from build123d import *

# Parameters (mm, degrees)
SKETCH1_W           = 5
SKETCH1_H           = 70
BOSS_EXTRUDE1_DEPTH = 10


with BuildPart() as part:
    # Sketch1 → Boss-Extrude1 (new body)
    with BuildSketch(Plane.XY):
        Polygon((-124.392981478, -115.783921891), (0, -115.783921891), (124.407018522, -115.783921891), (124.407018522, -15.783921891), (-0.05047515, -15.783921891), (-124.392981478, -15.783921891), align=None)
        with Locations((-31.092981478, -55.783921891)):
            Rectangle(SKETCH1_W, SKETCH1_H, mode=Mode.SUBTRACT)
        with Locations((-93.292981478, -55.783921891)):
            Rectangle(SKETCH1_W, SKETCH1_H, mode=Mode.SUBTRACT)
        with Locations((31.107018522, -55.783921891)):
            Rectangle(SKETCH1_W, SKETCH1_H, mode=Mode.SUBTRACT)
        with Locations((93.307018522, -55.783921891)):
            Rectangle(SKETCH1_W, SKETCH1_H, mode=Mode.SUBTRACT)
    extrude(amount=BOSS_EXTRUDE1_DEPTH)


solid = part.part
The listing builds one solid part. Answer for the finished solid, in the listing's coordinates (mm). A direction names the side the tool comes from. Round coordinates to 2 decimals unless told otherwise and drop trailing zeros. Write each loop counter-clockwise with the first axis right and the second up, starting at its lowest first coordinate (ties: lowest second). Pieces come first, ordered by that corner, then holes. Notation, with made-up numbers: M 17.5,34 L 57.5,34 A13 ccw 57.5,58 Z; hole C -36,-2.75 d10. An arc over 180 degrees is marked long. Write each question's results on one line, items separated by ' | '. Start each with the question number.
Item 1: The mould has two halves that part along X. Classify faces 1 (the flat face through (-2, -65, 10)), 2 (the flat face through (33.607, -56, 5)), 3 (the flat face through (-124.393, -65, 5)): +X half, -X half, draft (parallel to the pull), parting line (faces both ways), or undercut.
Item 2: Straight lines are drawn through the part: probe 1 along X at (y, z) = (-34.5, 3.5); probe 2 along Y at (x, z) = (95.5, 7.75). For each, find the intervals that lie inside material, in ascending order.
Item 3: Find section B-B on z = 8.25. Write down the section's boundary in (x, y), and give its area (3 significant figures).
Item 4: Find section A-A on y = -53.5. Write down the section's boundary in (x, z), and give its area (3 significant figures).
Item 5: Which of the six approach directions +Z, -Z, +X, -X, +Y, -Y give full straight-line access (tool end or side, diameter ignored) to faces 4 (the flat face through (93, -90.784, 5)), 5 (the flat face through (-2, -65, 0))?
Answer block:
1) face 1: draft | face 2: undercut | face 3: -X half
2) probe 1: x = -124.39 to -95.79, -90.79 to -33.59, -28.59 to 28.61, 33.61 to 90.81, 95.81 to 124.41 | probe 2: y = -115.78 to -90.78, -20.78 to -15.78
3) outline: M -124.39,-115.78 L 124.41,-115.78 L 124.41,-15.78 L -124.39,-15.78 Z; hole M -95.79,-90.78 L -90.79,-90.78 L -90.79,-20.78 L -95.79,-20.78 Z; hole M -33.59,-90.78 L -28.59,-90.78 L -28.59,-20.78 L -33.59,-20.78 Z; hole M 28.61,-90.78 L 33.61,-90.78 L 33.61,-20.78 L 28.61,-20.78 Z; hole M 90.81,-90.78 L 95.81,-90.78 L 95.81,-20.78 L 90.81,-20.78 Z | area: 23,500 mm²
4) outline: M -124.39,0 L -95.79,0 L -95.79,10 L -124.39,10 Z; M -90.79,0 L -33.59,0 L -33.59,10 L -90.79,10 Z; M -28.59,0 L 28.61,0 L 28.61,10 L -28.59,10 Z; M 33.61,0 L 90.81,0 L 90.81,10 L 33.61,10 Z; M 95.81,0 L 124.41,0 L 124.41,10 L 95.81,10 Z | area: 2,290 mm²
5) face 4: +Z, -Z | face 5: -Z, +X, -X, +Y, -Y
